The listing builds one solid part. Answer for the finished solid, in the listing's coordinates (mm). Give positions to 0.01 mm unless a question says otherwise; leave off trailing zeros. Loops run counter-clockwise (first coordinate to the right, second up) from the corner with the lowest first, then second, coordinate; pieces in that order, holes last. Notation, with made-up numbers: M 39.5,3 L 68.5,3 A28 ccw 68.5,29 Z; hole C -39.75,-23.75 d5. An arc over 180 degrees is marked long. One line per item, written item: value. Start each with the question number.
Q1. A cutting plane is placed at C-C, the plane y = 0. Determine the outline of the cut face in (x, z), and give its area (3 significant figures).
Q2. A cutting plane is placed at B-B, the plane x = -55. Determine the outline of the cut face in (y, z).
Q3. A cutting plane is placed at A-A, the plane x = 10. Determine the outline of the cut face in (y, z), and give its area (3 significant figures).
Q4. Flat-ended cylindrical pins translate along their axes: pin 1 (4 mm diameter, centred on x = -57, z = -2, fed in from +Y); pin 2 (5 mm diameter, centred on x = -59, z = 1, fed in from +Y). Find the tip coordinate at first contact, or state that the pin passes through.
Q5. A cutting plane is placed at D-D, the plane z = 0.5. Determine the outline of the cut face in (x, y), and give its area (3 significant figures).
Q6. Consider L1, parallel to Y at x = -55, z = 0.75; L2, parallel to Y at x = -52, z = -0.5; L3, parallel to Y at x = -46, z = 4.25. Determine where each line is inside the solid, lowest interval first.
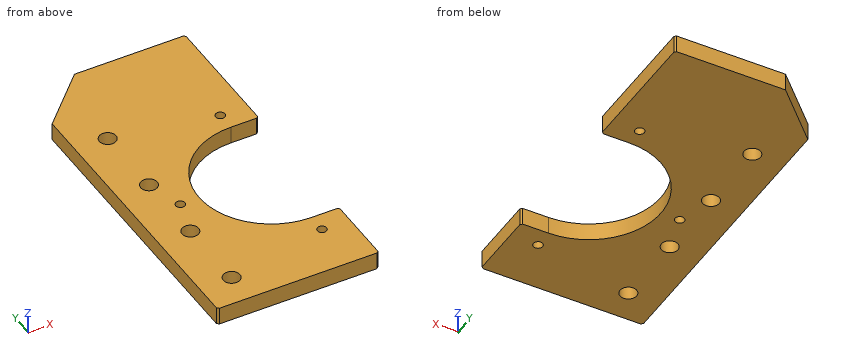
from build123d import *

# Parameters (mm, degrees)
BOSS_EXTRUDE1_DEPTH   = 4.7625
M8_CLEARANCE_HOLE1_D  = 9
M6X1_0_TAPPED_HOLE1_D = 5
CHAMFER1_SIZE         = 1


with BuildPart() as part:
    # Sketch1 → Boss-Extrude1 (new, symmetric)
    with BuildSketch(Plane.XY):
        with BuildLine():
            Line((0, -39), (15, -39))
            Line((15, -39), (15, -77.5))
            Line((15, -77.5), (-72.5, -77.5))
            Line((-72.5, -77.5), (-72.5, 82.5))
            Line((-72.5, 82.5), (-45, 110))
            Line((-45, 110), (15, 110))
            Line((15, 110), (15, 39))
            Line((15, 39), (0, 39))
            ThreePointArc((0, 39), (-39, 0), (0, -39))
        make_face()
    extrude(amount=BOSS_EXTRUDE1_DEPTH, both=True)

    # M8 Clearance Hole1 (through all)
    with Locations(Plane.XY.offset(4.7625)):
        with Locations((-55, 60), (-55, 20), (-55, -20), (-55, -60)):
            Hole(M8_CLEARANCE_HOLE1_D / 2)

    # M6x1.0 Tapped Hole1 (through all)
    with Locations(Plane.XY.offset(4.7625)):
        with Locations((0, 49.2125), (-49.2125, 0), (0, -49.2125)):
            Hole(M6X1_0_TAPPED_HOLE1_D / 2)

    # Chamfer1
    chamfer1_edges = [part.edges().sort_by_distance(p)[0] for p in [
        (15, -39, 0),
        (15, -77.5, 0),
        (-72.5, -77.5, 0),
        (15, 110, 0),
        (15, 39, 0),
    ]]
    chamfer(chamfer1_edges, length=CHAMFER1_SIZE)


solid = part.part
Answer block:
1. outline: M -72.5,-4.76 L -51.71,-4.76 L -51.71,4.76 L -72.5,4.76 Z; M -46.71,-4.76 L -39,-4.76 L -39,4.76 L -46.71,4.76 Z
1. area: 271 mm^2
2. outline: M -77.5,-4.76 L -64.5,-4.76 L -64.5,4.76 L -77.5,4.76 Z; M -55.5,-4.76 L -24.5,-4.76 L -24.5,4.76 L -55.5,4.76 Z; M -15.5,-4.76 L 15.5,-4.76 L 15.5,4.76 L -15.5,4.76 Z; M 24.5,-4.76 L 55.5,-4.76 L 55.5,4.76 L 24.5,4.76 Z; M 64.5,-4.76 L 100,-4.76 L 100,4.76 L 64.5,4.76 Z
3. outline: M -77.5,-4.76 L -39,-4.76 L -39,4.76 L -77.5,4.76 Z; M 39,-4.76 L 110,-4.76 L 110,4.76 L 39,4.76 Z
3. area: 1,040 mm^2
4. pin 1: y = 100
4. pin 2: y = 98.5
5. outline: M -72.5,-76.5 L -71.5,-77.5 L 14,-77.5 L 15,-76.5 L 15,-40 L 14,-39 L 0,-39 A39 cw 0,39 L 14,39 L 15,40 L 15,109 L 14,110 L -45,110 L -72.5,82.5 Z; hole C -55,-60 d9; hole C -55,-20 d9; hole C -55,20 d9; hole C -55,60 d9; hole C -49.21,0 d5; hole C 0,-49.21 d5; hole C 0,49.21 d5
5. area: 12,200 mm^2
6. L1: -77.5 to -64.5, -55.5 to -24.5, -15.5 to 15.5, 24.5 to 55.5, 64.5 to 100
6. L2: -77.5 to -63.35, -56.65 to -23.35, -16.65 to 16.65, 23.35 to 56.65, 63.35 to 103
6. L3: -77.5 to 109
